Geometry check sheet. Reference: drawing and pictorial views, mm from the part's lowest x, y, z. A direction names the side the tool comes from. Coordinates: 2 decimals unless noted, no trailing zeros. Write each loop counter-clockwise with the first axis right and the second up, starting at its lowest first coordinate (ties: lowest second). Pieces come first, ordered by that corner, then holes. Notation, with made-up numbers: M 47,-36 L 89,-36 A30 cw 89,-12 Z; hole C -23.75,33 d7. An arc over 180 degrees is marked long. One line per item, written item: value.
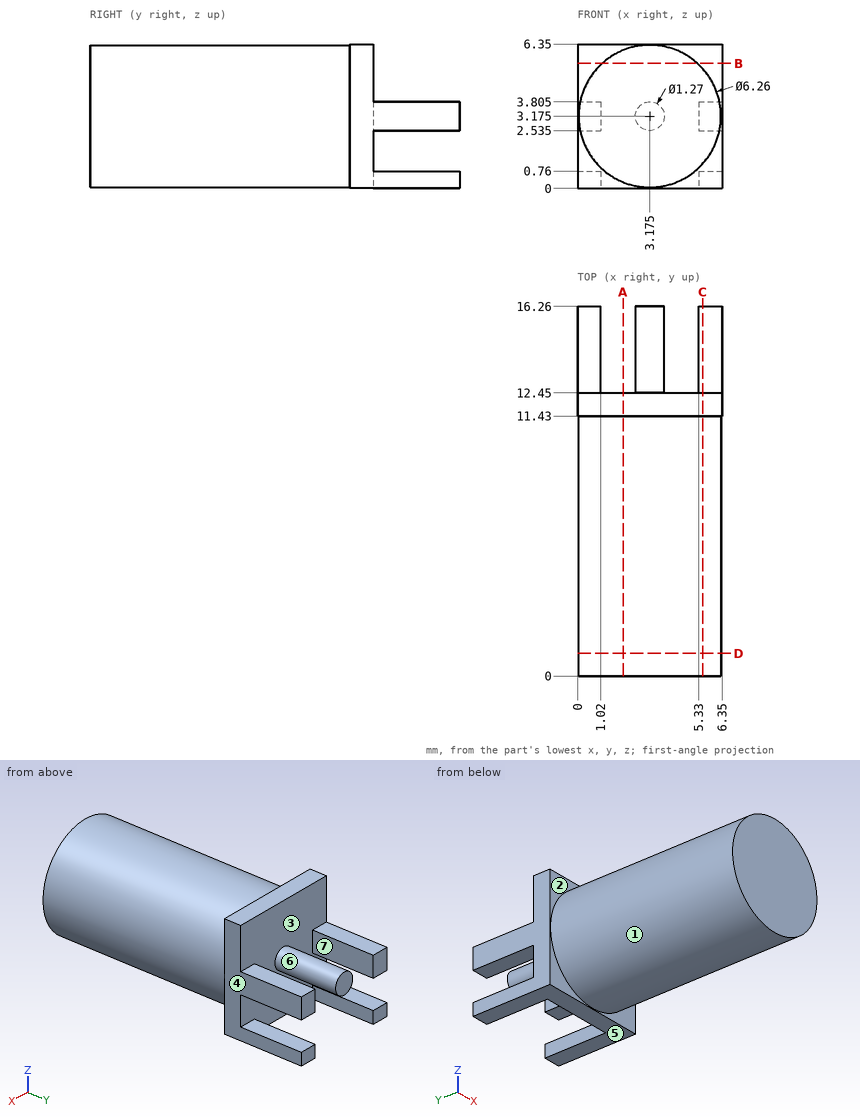
Item 1: Draft check along X on the marked faces 1, 2, 3 and 4. Enter one of: released by +X, released by -X, zero draft, split by the parting line, or undercut.
The answers:
face 1: split by the parting line
face 2: zero draft
face 3: undercut
face 4: released by +X
Item 2: Cross-section at A-A, the plane x = 2. Enter the section's corners in (y, z).
The answers:
outline: M 0,0.27 L 11.43,0.27 L 11.43,0 L 12.45,0 L 12.45,6.35 L 11.43,6.35 L 11.43,6.08 L 0,6.08 Z
Item 3: Cross-section at B-B, the plane z = 5.5. Enter the section's corners in (x, y).
The answers:
outline: M 0,11.43 L 1.08,11.43 L 1.08,0 L 5.27,0 L 5.27,11.43 L 6.35,11.43 L 6.35,12.45 L 0,12.45 Z
Item 4: Cross-section at D-D, the plane y = 1. Enter the section's corners in (x, z) (3 decimals), and give its area (3 significant figures).
The answers:
outline: C 3.175,3.175 d6.26
area: 30.8 mm²
Item 5: Scan lines: line 1 (X direction, y = 12.5, z = 2.75); line 2 (Z direction, x = 6, y = 13) (3 decimals); line 3 (X direction, y = 14.75, z = 3). Record each from-to range of solid material in increasing order.
The answers:
line 1: x = 0 to 1.02, 2.7 to 3.65, 5.33 to 6.35
line 2: z = 0 to 0.76, 2.535 to 3.805
line 3: x = 0 to 1.02, 2.56 to 3.79, 5.33 to 6.35
Item 6: Go/stop test with flat-tipped pins: P1, Ø1.5, axis at x = 2, y = 14, coming from the +Z side; P2, Ø1.1, axis at x = 0.5, y = 14, coming from the +Z side (3 decimals); P3, Ø2, axis at y = 4, z = 3, coming from the -X side (3 decimals). Record where each tip stops, or that it passes through.
The answers:
P1: stops at z = 3.65
P2: stops at z = 3.805
P3: stops at x = 0.045
Item 7: Cross-section at C-C, the plane x = 5.5. Enter the section's corners in (y, z) (3 decimals), and give its area (3 significant figures).
The answers:
outline: M 0,1.079 L 11.43,1.079 L 11.43,0 L 16.26,0 L 16.26,0.76 L 12.45,0.76 L 12.45,2.535 L 16.26,2.535 L 16.26,3.805 L 12.45,3.805 L 12.45,6.35 L 11.43,6.35 L 11.43,5.271 L 0,5.271 Z
area: 62.1 mm²
Item 8: Access from +Z, -Z, +X, -X, +Y, -Y to the whole of each face (thin tool, end or side, straight path). Record for the marked faces 5, 6 and 7.
The answers:
face 5: -Z, +X, -X, +Y, -Y
face 6: +Y
face 7: +Z, -Z, +Y
